```python
from build123d import *

# Parameters (mm, degrees)
BOSS_EXTRUDE1_DEPTH = 2
SKETCH2_R           = 0.75
CUT_EXTRUDE1_DEPTH  = 15.121858943
BOSS_EXTRUDE2_START = 2
SKETCH4_R           = 3.63
SKETCH4_R_2         = 2.88
BOSS_EXTRUDE2_DEPTH = 2


with BuildPart() as part:
    # Sketch1 → Boss-Extrude1 (new body)
    with BuildSketch(Plane(origin=(0, 0, 0), x_dir=(1, 0, 0), z_dir=(0, 1, 0))):
        with BuildLine():
            Line((-12.26625, 1.476181201), (-0.644325, 3.572358506))
            ThreePointArc((-0.644325, 3.572358506), (0.003746369, 3.629998067), (0.651697383, 3.571020935))
            Line((0.651697383, 3.571020935), (12, 1.5))
            ThreePointArc((12, 1.5), (13.494033434, 0.133656648), (12.26625, -1.476181201))
            Line((12.26625, -1.476181201), (0.644325, -3.572358506))
            ThreePointArc((0.644325, -3.572358506), (0, -3.63), (-0.644325, -3.572358506))
            Line((-0.644325, -3.572358506), (-12.26625, -1.476181201))
            ThreePointArc((-12.26625, -1.476181201), (-13.5, 0), (-12.26625, 1.476181201))
        make_face()
    extrude(amount=BOSS_EXTRUDE1_DEPTH)

    # Sketch2 → Cut-Extrude1 (cut, through all)
    with BuildSketch(Plane(origin=(0, 2, 0), x_dir=(1, 0, 0), z_dir=(0, 1, 0))):
        with Locations(Location((12, 0, 0), (0, 0, 270))):
            Circle(SKETCH2_R)
        with Locations(Location((9, 0, 0), (0, 0, 270))):
            Circle(SKETCH2_R)
        with Locations(Location((6, 0, 0), (0, 0, 270))):
            Circle(SKETCH2_R)
    cut_extrude1 = extrude(amount=-CUT_EXTRUDE1_DEPTH, mode=Mode.SUBTRACT)

    # Mirror1: Cut-Extrude1 across plane
    add(cut_extrude1.mirror(Plane(origin=(0, 0, 0), x_dir=(0, 0, 1), z_dir=(1, 0, 0))), mode=Mode.SUBTRACT)

    # Sketch4 → Boss-Extrude2 (add)
    with BuildSketch(Plane.XZ.offset(BOSS_EXTRUDE2_START)):
        with Locations(Location((0, 0, 0), (0, 0, 270))):
            Circle(SKETCH4_R)
        with Locations(Location((0, 0, 0), (0, 0, 270))):
            Circle(SKETCH4_R_2, mode=Mode.SUBTRACT)
    extrude(amount=-BOSS_EXTRUDE2_DEPTH)


solid = part.part
```
Input: part model. Units: mm. Frame: model coordinates. A direction names the side the tool comes from. Coordinates: 2 decimals unless noted, no trailing zeros. Loops run counter-clockwise (first coordinate to the right, second up) from the corner with the lowest first, then second, coordinate; pieces in that order, holes last.
Q1. Section A-A, the plane y = 0.3. Return the cut outline in (x, z).
Results are:
outline: (-12.27, -1.48) - (-0.64, -3.57) arc R3.63 ccw to (0.65, -3.57) - (12, -1.5) arc R1.5 ccw to (12.27, 1.48) - (0.64, 3.57) arc R3.63 ccw to (-0.64, 3.57) - (-12.27, 1.48) arc R1.5 ccw to start; hole circle Ø1.5 at (-12, 0); hole circle Ø1.5 at (-9, 0); hole circle Ø1.5 at (-6, 0); hole circle Ø1.5 at (6, 0); hole circle Ø1.5 at (9, 0); hole circle Ø1.5 at (12, 0)
Q2. Section D-D, the plane z = 1. Return the cut outline in (x, y), and give its area (3 significant figures).
Results are:
outline: (-13.12, 0) - (-3.49, 0) - (-3.49, -2) - (-2.7, -2) - (-2.7, 0) - (2.7, 0) - (2.7, -2) - (3.49, -2) - (3.49, 0) - (13.12, 0) - (13.12, 2) - (-13.12, 2) - close
area: 55.6 mm2
Q3. Section C-C, the plane z = 0. Give the number of separate pieces and of enclosed holes in the cut face, and give its area (3 significant figures).
Results are:
separate pieces: 7
enclosed holes: 0
area: 39.0 mm2
Q4. Contact query for flat-ended pins moving along their axis: pin 1 (2.5 mm diameter, centred on x = -9, z = 0, fed in from -Y); pin 2 (1.5 mm diameter, centred on y = 1.5, z = 1.5, fed in from +X); pin 3 (1.5 mm diameter, centred on x = 2.5, y = 1, fed in from +Z). Output: stop coordinate, or through.
Results are:
pin 1: stops at y = 0
pin 2: stops at x = 13.3
pin 3: stops at z = 3.37
Q5. Set-up query: faces 4 (the flat face through (0, 0, 0)), 5 (the flat face through (3, -2, 1)). Return all of +Z, -Z, +X, -X, +Y, -Y with unobstructed straight access to the full face (end or side cutting, diameter ignored); none if empty.
Results are:
face 4: -Y
face 5: +Z, -Z, +X, -X, -Y
Q6. Line query: line 1 along X through (y, z) = (-1, 0); line 2 along Y through (x, z) = (2, 1.5); line 3 along Z through (x, y) = (0.75, -1.25). Output: solid intervals per line, ascending.
Results are:
line 1: x = -3.63 to -2.88, 2.88 to 3.63
line 2: y = 0 to 2
line 3: z = -3.55 to -2.78, 2.78 to 3.55
Q7. Section B-B, the plane x = -12. Return the cut outline in (y, z).
Results are:
outline: (0, -1.52) - (2, -1.52) - (2, -0.75) - (0, -0.75) - close; (0, 0.75) - (2, 0.75) - (2, 1.52) - (0, 1.52) - close
Q8. Mould query, pull axis Z, two halves, no side actions, for faces 1 (the cylindrical face through (-13.5, 1, 0)), 2 (the cylindrical face through (9.632, 1.014, 0.403)), 3 (the flat face through (-6.37, 0.99, 2.54)). Classes: +Z half, -Z half, draft (parallel to the pull), parting line (faces both ways), or undercut.
Results are:
face 1: parting line
face 2: undercut
face 3: +Z half
